Autodesk Inventor part; units mm, degrees
ref_plane "YZ Plane" through (0, 0, 0) normal (1, 0, 0) x (0, 1, 0)
ref_plane "XZ Plane" through (0, 0, 0) normal (0, 1, 0) x (-1, 0, 0)
ref_plane "XY Plane" through (0, 0, 0) normal (0, 0, 1) x (1, 0, 0)
sketch "Sketch1" plane through (0, 0, 0) normal (0, 0, 1) x (1, 0, 0)
  circle A0 centre (0.25, 36.05) radius 30
  line L0 (-21, -56.05) -> (-21, -1.05)
  line L1 (-21, -1.05) -> (21.5, -1.05)
  line L2 (21.5, -1.05) -> (21.5, -56.05)
  line L3 (21.5, -56.05) -> (-21, -56.05)
  arc A1 (-41, -66.05) -> (-36, -71.05) centre (-36, -66.05) ccw
  line L4 (-36, -71.05) -> (36, -71.05)
  arc A2 (36, -71.05) -> (41, -66.05) centre (36, -66.05) ccw
  line L5 (41, -66.05) -> (41, 71.05)
  line L6 (41, 71.05) -> (-41, 71.05)
  line L7 (-41, 71.05) -> (-41, -66.05)
  circle A3 centre (-36, 66.05) radius 3.25
  circle A4 centre (-36, -66.05) radius 3.25
  circle A5 centre (36, 66.05) radius 3.25
  circle A6 centre (36, -66.05) radius 3.25
  circle A7 centre (0.25, 36.05) radius 3.75
  point P0 (0, 0)
  dimension "d0" = 60
extrude "Extrusion1" add sketch "Sketch1" along normal blind 9 contours A0 | A7
sketch "Sketch2" plane through (0.25, 36.05, 0) normal (0, 0, -1) x (-1, 0, 0)
  circle A0 centre (0, 0) radius 3.15
  line L0 (-1.65, 2.6833) -> (-1.65, -2.6833)
  circle A1 centre (0, 0) radius 30
  point P0 (0.25, -36.05)
  dimension "d5" = 6.3
  dimension "d6" = 4.8
  dimension "d7" = 0
extrude "Extrusion2" cut sketch "Sketch2" against normal blind 7 contours A0 L0 picked at (1.6001, 0.6823)
sketch "Sketch3" plane through (0.25, 36.05, 0) normal (0, 0, -1) x (-1, 0, 0)
  circle A0 centre (0, 0) radius 3.15
  circle A1 centre (0, 0) radius 7.5
  circle A2 centre (0, 0) radius 25
  circle A3 centre (0, 0) radius 30
  point P0 (0.25, -36.05)
  dimension "d10" = 15
  dimension "d11" = 5
  dimension "d12" = 26.85
  dimension "d13" = 6.3
extrude "Extrusion3" cut sketch "Sketch3" against normal blind 7 contours A2
sketch "Sketch4" plane through (0.25, 36.05, 0) normal (0, 0, -1) x (-1, 0, 0)
  circle A0 centre (0, 0) radius 30
  circle A1 centre (0, 0) radius 25
  point P0 (0.25, -36.05)
extrude "Extrusion4" add sketch "Sketch4" along normal blind 6
properties part number "knob"
Could you check a few things on this model? Use its own coordinates, in mm. A direction names the side the tool comes from. Round coordinates to 2 decimals unless told otherwise and drop trailing zeros. Order: outer loops, then holes, each group sorted by start corner. A loop starts at its lowest first (then second) coordinate and runs counter-clockwise, first axis right, second up.
(1) Imagine slicing it at A-A (z = 5.5). Write out the boundary of the cut face in (x, y).
Response values:
outline: circle Ø60 at (0.25, 36.05); circle Ø15 at (0.25, 36.05); hole circle Ø50 at (0.25, 36.05); hole (1.9, 33.37) - (1.9, 38.73) arc R3.15 ccw (long way) to start
(2) Which directions (+Z, -Z, +X, -X, +Y, -Y) give clear straight access to the entire face, cutting with the end or side of a thin tool? Please do faces 3 (the flat face through (7, 61, -6)), 4 (the cylindrical face through (1.88, 28.73, 3.45)).
Response values:
face 3: -Z, +X, -X, +Y, -Y
face 4: -Z
(3) If we mould it in two halves opening along X, with no side actions, what happens to faces 1 (the flat face through (0, 36, 9)), 2 (the flat face through (1.9, 36, 3))? For each: released by +X, released by -X, zero draft, split by the parting line, or undercut.
Response values:
face 1: zero draft
face 2: undercut
(4) Please list where these lines run through material, in increasing order: line 1 along Y through (x, z) = (0.25, 4.25); line 2 along Y through (x, z) = (2, 0.25); line 3 along Z through (x, y) = (21.5, 40).
Response values:
line 1: y = 6.05 to 11.05, 28.55 to 32.9, 39.2 to 43.55, 61.05 to 66.05
line 2: y = 6.1 to 11.11, 28.76 to 43.34, 60.99 to 66
line 3: z = 7 to 9
(5) Imagine slicing it at B-B (x = -1). Write out the boundary of the cut face in (y, z).
Response values:
outline: (6.08, -6) - (11.08, -6) - (11.08, 7) - (28.65, 7) - (28.65, 0) - (33.16, 0) - (33.16, 7) - (38.94, 7) - (38.94, 0) - (43.45, 0) - (43.45, 7) - (61.02, 7) - (61.02, -6) - (66.02, -6) - (66.02, 9) - (6.08, 9) - close
(6) Imagine slicing it at D-D (z = -1.5). Write out the boundary of the cut face in (x, y), plus the area to 3 significant figures.
Response values:
outline: circle Ø60 at (0.25, 36.05); hole circle Ø50 at (0.25, 36.05)
area: 864 mm2
(7) I'm going to push flat-ended pins straight in: pin 1 (6 mm diameter, centred on y = 22.5, z = -0.5, fed in from -X); pin 2 (1.6 mm diameter, centred on y = 35, z = 3, fed in from -X); pin 3 (2 mm diameter, centred on x = 0, y = 54, fed in from -Z). Where does each tip first touch, or does it pass through?
Response values:
pin 1: stops at x = -27.83
pin 2: stops at x = -29.75
pin 3: stops at z = 7
(8) Imagine slicing it at C-C (y = 36.05). Write out the boundary of the cut face in (x, z).
Response values:
outline: (-29.75, -6) - (-24.75, -6) - (-24.75, 7) - (-7.25, 7) - (-7.25, 0) - (-2.9, 0) - (-2.9, 7) - (1.9, 7) - (1.9, 0) - (7.75, 0) - (7.75, 7) - (25.25, 7) - (25.25, -6) - (30.25, -6) - (30.25, 9) - (-29.75, 9) - close
